Autodesk Inventor part; units mm, degrees
ref_plane "YZ Plane" through (0, 0, 0) normal (1, 0, 0) x (0, 1, 0)
ref_plane "XZ Plane" through (0, 0, 0) normal (0, 1, 0) x (-1, 0, 0)
ref_plane "XY Plane" through (0, 0, 0) normal (0, 0, 1) x (1, 0, 0)
sketch "Sketch1" plane through (0, 0, 0) normal (0, 0, 1) x (1, 0, 0)
  line L0 (0, 0) -> (0, 4)
  line L1 (0, 4) -> (4.5, 4)
  line L2 (4.5, 4) -> (4.5, 5)
  line L3 (4.5, 5) -> (12.9, 5)
  line L4 (12.9, 5) -> (12.9, 6)
  line L5 (120.5, 6) -> (120.5, 5)
  line L6 (120.5, 5) -> (128.9, 5)
  line L7 (128.9, 5) -> (128.9, 4)
  line L8 (128.9, 4) -> (133.4, 4)
  line L9 (133.4, 4) -> (133.4, 0)
  line L10 (133.4, 0) -> (0, 0)
  line L11 (66.7, 6) -> (66.7, 0) construction
  line L12 (12.9, 6) -> (17.9, 6)
  line L13 (17.9, 6) -> (17.9, 5)
  line L14 (17.9, 5) -> (115.5, 5)
  line L15 (115.5, 5) -> (115.5, 6)
  line L16 (115.5, 6) -> (120.5, 6)
  dimension "d0" = 4
  dimension "d1" = 5
  dimension "d3" = 4.5
  dimension "d4" = 107.6
  dimension "d5" = 124.4
  dimension "d6" = 4.5
  dimension "d8" = 5
  dimension "d9" = 5
  dimension "d11" = 6
revolve "Revolution1" add sketch "Sketch1" angle 360 about axis through (133.4, 0, 0) along (-1, 0, 0)
properties part number "Stopper Axle" material "Stainless Steel"
For this review, take the finished solid that the model builds, in its own axes (mm). A direction names the side the tool comes from. Round coordinates to 2 decimals unless told otherwise and drop trailing zeros. Loops run counter-clockwise (first coordinate to the right, second up) from the corner with the lowest first, then second, coordinate; pieces in that order, holes last.
Q1. Add section A-A on y = 0. Write out the cut boundary in (x, z), plus the area to 3 significant figures.
Result sheet:
outline: (0, -4) - (4.5, -4) - (4.5, -5) - (12.9, -5) - (12.9, -6) - (17.9, -6) - (17.9, -5) - (115.5, -5) - (115.5, -6) - (120.5, -6) - (120.5, -5) - (128.9, -5) - (128.9, -4) - (133.4, -4) - (133.4, 4) - (128.9, 4) - (128.9, 5) - (120.5, 5) - (120.5, 6) - (115.5, 6) - (115.5, 5) - (17.9, 5) - (17.9, 6) - (12.9, 6) - (12.9, 5) - (4.5, 5) - (4.5, 4) - (0, 4) - close
area: 1,340 mm2
Q2. Add section C-C on x = 41. Write out the cut boundary in (y, z).
Result sheet:
outline: circle Ø10 at (0, 0)
Q3. To check wall thickness, follow line 1 along X through (y, z) = (-3.75, -4); line 2 along X through (y, z) = (3.5, -3.5); line 3 along Z through (x, y) = (18, -3). State the ranges of each line that lie inside material, in increasing order.
Result sheet:
line 1: x = 12.9 to 17.9, 115.5 to 120.5
line 2: x = 4.5 to 128.9
line 3: z = -4 to 4
Q4. Insertion check: pin 1 Ø3 at (x, z) = (82.5, 1) entering from +Y; pin 2 Ø1.5 at (y, z) = (-4.5, -4) entering from +X; pin 3 Ø3 at (x, y) = (109.5, -2) entering from +Z. Each pin has a flat end and moves straight along its axis. Give the tip position at first contact, or say it passes through.
Result sheet:
pin 1: stops at y = 5
pin 2: stops at x = 120.5
pin 3: stops at z = 4.97
Q5. Mouldability with a two-part tool opening along X and no side actions: class faces 1 (the face through (8.76, -1.08, -4.88)), 2 (the face through (120.5, -4, -4)), 3 (the face through (0, 0, 0)), 4 (the face through (17.9, -4, -4)) as +X half, -X half, draft (parallel to the pull), parting line (faces both ways), or undercut.
Result sheet:
face 1: draft
face 2: +X half
face 3: -X half
face 4: undercut
Q6. Machinability: for faces 5 (the face through (115.5, -4, -4)), 6 (the face through (12.9, -4, -4)), 7 (the face through (131.182, -0.867, -3.905)), which of the approach directions +Z, -Z, +X, -X, +Y, -Y give a long, thin tool a straight path to every point of the face, cutting with its end or side? Answer none if there is none.
Result sheet:
face 5: none
face 6: -X
face 7: +X
